Geometry check sheet. Reference: the model listing, model coordinates, mm. Face numbers are marked on the shaded views. Round coordinates to 2 decimals unless told otherwise and drop trailing zeros. Order: outer loops, then holes, each group sorted by start corner. A loop starts at its lowest first (then second) coordinate and runs counter-clockwise, first axis right, second up.
(1) Sectioned sample at A-A (z = -2.3). Record the boundary of the cut face in (x, y).
(2) Go/stop test with flat-tipped pins: pin 1 (1.5 mm diameter, centred on x = 2, z = -3, fed in from +Y); pin 2 (1 mm diameter, centred on x = -1.5, y = -1.5, fed in from -Z); pin 3 (4 mm diameter, centred on x = 0, y = 0, fed in from -Z). Record where each tip stops, or that it passes through.
(3) Release check for a two-part mould opening along Y. For the marked faces 1, 2 and 3 record: +Y half, -Y half, draft (parallel to the pull), parting line (faces both ways), or undercut.
(4) Material ranges on line 1 along Y through (x, z) = (-0.75, -1.35); line 2 along Y through (x, z) = (-1.5, -1.1); line 3 along X through (y, z) = (0.5, -2.05), recorded low to high.
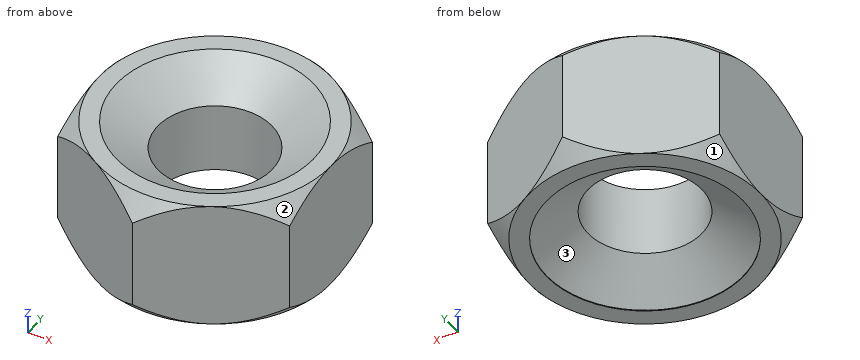
from build123d import *

# Parameters (mm, degrees)
THREADSCHEMATIC_START     = -4.1402
THREADSCHEMATIC_OUTLINE_R = 1.8415
THREADSCHEMATIC_DEPTH     = 4.1402


# Read off the part's stored shape, not the designer's step: ThreadSchematic
with BuildPart() as part:
    # ThreadSchematic outline → ThreadSchematic (new body)
    with BuildSketch(Plane.XY.offset(THREADSCHEMATIC_START)):
        Polygon((3.7465, 2.163042784), (0, 4.326085567), (-3.7465, 2.163042784), (-3.7465, -2.163042784), (0, -4.326085567), (3.7465, -2.163042784), align=None)
        Circle(THREADSCHEMATIC_OUTLINE_R, mode=Mode.SUBTRACT)
    extrude(amount=THREADSCHEMATIC_DEPTH)

    # Sketch3 → Double-Chamfer (revolve, cut)
    with BuildSketch(Plane(origin=(0, 0, 0), x_dir=(0, 0, -1), z_dir=(1, 0, 0))):
        Polygon((4.1402, 3.7465), (3.5052, 4.326085567), (3.5052, 17.026085567), (16.8402, 17.026085567), (16.8402, 3.7465), align=None)
        Polygon((0.635, 17.026085567), (-12.7, 17.026085567), (-12.7, 3.7465), (0, 3.7465), (0.635, 4.326085567), align=None)
    revolve(axis=Axis((0, 0, 0), (0, 0, -1)), mode=Mode.SUBTRACT)

    # EndChamferSke → EndChamfer (revolve, cut)
    with BuildSketch(Plane(origin=(0, 0, 0), x_dir=(0, 0, -1), z_dir=(1, 0, 0)), mode=Mode.PRIVATE) as endchamfer_sk:
        Polygon((4.1148, 3.175), (3.087700573, 1.70815), (4.1656, 1.70815), (4.1656, 3.175), align=None)
        Polygon((-0.0508, 3.175), (0, 3.175), (1.027099427, 1.70815), (-0.0508, 1.70815), align=None)
    revolve(endchamfer_sk.sketch.rotate(Axis((0, 0, -25.037505729), (0, 0, -1)), 90), axis=Axis((0, 0, -25.037505729), (0, 0, -1)), mode=Mode.SUBTRACT)


solid = part.part
Answer below:
1. outline: (-3.75, -2.16) - (0, -4.33) - (3.75, -2.16) - (3.75, 2.16) - (0, 4.33) - (-3.75, 2.16) - close; hole circle Ø3.68 at (0, 0)
2. pin 1: stops at y = 3.6
2. pin 2: stops at z = -3.73
2. pin 3: stops at z = -3.29
3. face 1: +Y half
3. face 2: -Y half
3. face 3: undercut
4. line 1: y = -3.89 to -1.68, 1.68 to 3.89
4. line 2: y = -3.46 to -1.07, 1.07 to 3.46
4. line 3: x = -3.75 to -1.77, 1.77 to 3.75
